from build123d import *

# Parameters (mm, degrees)
SKETCH1_W           = 42
SKETCH1_H           = 42
BOSS_EXTRUDE1_DEPTH = 37.5
SKETCH2_R           = 2.5
BOSS_EXTRUDE2_DEPTH = 23
SKETCH3_R           = 1.5
CUT_EXTRUDE1_DEPTH  = 8
SKETCH4_R           = 11
BOSS_EXTRUDE3_DEPTH = 3
CHAMFER1_SIZE       = 4
SKETCH5_W           = 18
SKETCH5_H           = 10
BOSS_EXTRUDE4_DEPTH = 6
FILLET1_START       = 10
FILLET1_DEPTH       = 19.5
FILLET2_START       = 10
FILLET2_DEPTH       = 19.5
FILLET3_START       = 10
FILLET3_DEPTH       = 19.5


with BuildPart() as part:
    # Sketch1 → Boss-Extrude1 (new body)
    with BuildSketch(Plane(origin=(0, 0, 0), x_dir=(1, 0, 0), z_dir=(0, 1, 0))):
        with Locations((21, 21)):
            Rectangle(SKETCH1_W, SKETCH1_H)
    extrude(amount=BOSS_EXTRUDE1_DEPTH)

    # Sketch2 → Boss-Extrude2 (add)
    with BuildSketch(Plane(origin=(0, 37.5, 0), x_dir=(1, 0, 0), z_dir=(0, 1, 0))):
        with Locations(Location((21, 21, 0), (0, 0, 90))):
            Circle(SKETCH2_R)
    extrude(amount=BOSS_EXTRUDE2_DEPTH)

    # Sketch3 → Cut-Extrude1 (cut)
    with BuildSketch(Plane(origin=(0, 37.5, 0), x_dir=(1, 0, 0), z_dir=(0, 1, 0))):
        with Locations(Location((6, 36, 0), (0, 0, 270))):
            Circle(SKETCH3_R)
        with Locations(Location((36, 36, 0), (0, 0, 270))):
            Circle(SKETCH3_R)
        with Locations(Location((36, 6, 0), (0, 0, 270))):
            Circle(SKETCH3_R)
        with Locations(Location((6, 6, 0), (0, 0, 270))):
            Circle(SKETCH3_R)
    extrude(amount=-CUT_EXTRUDE1_DEPTH, mode=Mode.SUBTRACT)

    # Sketch4 → Boss-Extrude3 (add)
    with BuildSketch(Plane(origin=(0, 37.5, 0), x_dir=(1, 0, 0), z_dir=(0, 1, 0))):
        with Locations(Location((21, 21, 0), (0, 0, 90))):
            Circle(SKETCH4_R)
    extrude(amount=BOSS_EXTRUDE3_DEPTH)

    # Chamfer1
    chamfer1_edges = [part.edges().sort_by_distance(p)[0] for p in [
        (0, 18.75, -42),
        (42, 18.75, -42),
        (42, 18.75, 0),
        (0, 18.75, 0),
    ]]
    chamfer(chamfer1_edges, length=CHAMFER1_SIZE)

    # Sketch5 → Boss-Extrude4 (add)
    with BuildSketch(Plane.ZY):
        with Locations((-21, 5)):
            Rectangle(SKETCH5_W, SKETCH5_H)
    extrude(amount=BOSS_EXTRUDE4_DEPTH)

    # Fillet1: read off the stored shape, not the designer's step
    # Fillet1 outline → Fillet1 (cut)
    with BuildSketch(Plane(origin=(0, 0, 0), x_dir=(1, 0, 0), z_dir=(0, 1, 0)).offset(FILLET1_START)):
        with BuildLine():
            ThreePointArc((42, 6.485281374), (41.543277195, 4.18918078), (40.242640687, 2.242640687))
            Line((40.242640687, 2.242640687), (42, 4))
            Line((42, 4), (42, 6.485281374))
        make_face()
        with BuildLine():
            ThreePointArc((39.757359313, 1.757359313), (37.81081922, 0.456722805), (35.514718626, 0))
            Line((35.514718626, 0), (38, 0))
            Line((38, 0), (39.757359313, 1.757359313))
        make_face()
    extrude(amount=FILLET1_DEPTH, mode=Mode.SUBTRACT)

    # Fillet2: read off the stored shape, not the designer's step
    # Fillet2 outline → Fillet2 (cut)
    with BuildSketch(Plane(origin=(0, 0, 0), x_dir=(1, 0, 0), z_dir=(0, 1, 0)).offset(FILLET2_START)):
        with BuildLine():
            ThreePointArc((35.514718626, 42), (37.81081922, 41.543277195), (39.757359313, 40.242640687))
            Line((39.757359313, 40.242640687), (38, 42))
            Line((38, 42), (35.514718626, 42))
        make_face()
        with BuildLine():
            ThreePointArc((40.242640687, 39.757359313), (41.543277195, 37.81081922), (42, 35.514718626))
            Line((42, 35.514718626), (42, 38))
            Line((42, 38), (40.242640687, 39.757359313))
        make_face()
    extrude(amount=FILLET2_DEPTH, mode=Mode.SUBTRACT)

    # Fillet3: read off the stored shape, not the designer's step
    # Fillet3 outline → Fillet3 (cut)
    with BuildSketch(Plane(origin=(0, 0, 0), x_dir=(1, 0, 0), z_dir=(0, 1, 0)).offset(FILLET3_START)):
        with BuildLine():
            ThreePointArc((6.485281374, 0), (4.18918078, 0.456722805), (2.242640687, 1.757359313))
            Line((2.242640687, 1.757359313), (4, 0))
            Line((4, 0), (6.485281374, 0))
        make_face()
        with BuildLine():
            ThreePointArc((1.757359313, 2.242640687), (0.456722805, 4.18918078), (0, 6.485281374))
            Line((0, 6.485281374), (0, 4))
            Line((0, 4), (1.757359313, 2.242640687))
        make_face()
        with BuildLine():
            ThreePointArc((0, 35.514718626), (0.456722805, 37.81081922), (1.757359313, 39.757359313))
            Line((1.757359313, 39.757359313), (0, 38))
            Line((0, 38), (0, 35.514718626))
        make_face()
        with BuildLine():
            ThreePointArc((2.242640687, 40.242640687), (4.18918078, 41.543277195), (6.485281374, 42))
            Line((6.485281374, 42), (4, 42))
            Line((4, 42), (2.242640687, 40.242640687))
        make_face()
    extrude(amount=FILLET3_DEPTH, mode=Mode.SUBTRACT)


solid = part.part
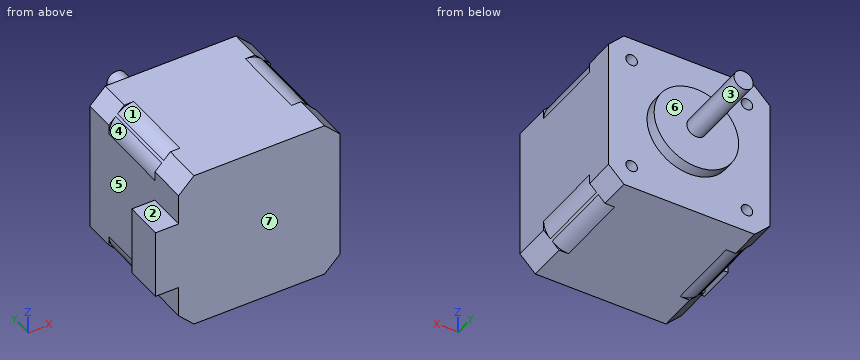
Here's how the part is built. I have some questions about the finished solid (model axes, mm). Face numbers are marked on the shaded views. A direction names the side the tool comes from. Give positions to 0.01 mm unless a question says otherwise; leave off trailing zeros. Loops run counter-clockwise (first coordinate to the right, second up) from the corner with the lowest first, then second, coordinate; pieces in that order, holes last. Notation, with made-up numbers: (-17.5, 79.25) -> (-10.5, 79.25) arc R28 cw to (-10.5, 116.25) -> close; hole circle Ø11 at (70.25, 63). An arc over 180 degrees is marked (long way). Answer as a JSON object with one key per item and string values. Group by question number.
Item 1: Imagine slicing it at A-A on x = 21. Write out the boundary of the cut face in (y, z).
Item 2: Imagine slicing it at B-B on y = 34. Write out the boundary of the cut face in (x, z), then the cut area to 3 significant figures.
Item 3: Imagine slicing it at C-C on z = -21. Write out the boundary of the cut face in (x, y).
Item 4: Thinking about a two-plate mould opening in Y: for the marked faces 4, 5, 6 and 7, which applies, pulls with the +Y half, pulls with the -Y half, needs draft (parallel to the pull), parting line crosses it, or undercut?
Item 5: On a 3-axis mill with a long thin cutter (end or side, diameter ignored), from which of +Z, -Z, +X, -X, +Y, -Y can I reach the whole of each face in a straight line? I mean the marked faces 1, 2 and 3. Say none if no direction works.
Item 6: I need wall thicknesses on L1, parallel to X at y = 32.75, z = -36; L2, parallel to X at y = 24.5, z = -20; L3, parallel to Y at x = 8.5, z = -20. Which ranges of each line are inside material? Lowest first, please.
Item 7: Imagine slicing it at D-D on y = 25. Write out the boundary of the cut face in (x, z), then the cut area to 3 significant figures.
Item 8: Will these pins go through, and if not, where does the flat tip stop? pin 1 (1.9 mm diameter, centred on x = 41.5, z = -38.5, fed in from +Y); pin 2 (21 mm diameter, centred on x = 11.5, z = -10.5, fed in from +Y); pin 3 (1.5 mm diameter, centred on x = 36, z = -36, fed in from +Y); pin 4 (12 mm diameter, centred on x = 12, y = 51, fed in from +Z).
Answer list:
{
 "1": {"outline": "(0, -42) -> (37.5, -42) -> (37.5, -32) -> (40.5, -32) -> (40.5, -23.5) -> (60.5, -23.5) -> (60.5, -18.5) -> (40.5, -18.5) -> (40.5, -10) -> (37.5, -10) -> (37.5, 0) -> (0, 0) -> close"},
 "2": {"outline": "(0, -38) -> (4, -42) -> (38, -42) -> (42, -38) -> (42, -4) -> (38, 0) -> (4, 0) -> (0, -4) -> close; hole circle Ø3 at (6, -36); hole circle Ø3 at (6, -6); hole circle Ø3 at (36, -36); hole circle Ø3 at (36, -6)", "area": "1,700 mm2"},
 "3": {"outline": "(-6, 0) -> (42, 0) -> (42, 37.5) -> (32, 37.5) -> (32, 40.5) -> (23.5, 40.5) -> (23.5, 60.5) -> (18.5, 60.5) -> (18.5, 40.5) -> (10, 40.5) -> (10, 37.5) -> (0, 37.5) -> (0, 10) -> (-6, 10) -> close"},
 "4": {"face 4": "undercut", "face 5": "needs draft", "face 6": "pulls with the +Y half", "face 7": "pulls with the -Y half"},
 "5": {"face 1": "+Z, -X", "face 2": "+Z, -X, +Y, -Y", "face 3": "+Y"},
 "6": {"L1": "x = 0 to 4.5, 7.5 to 34.5, 37.5 to 42", "L2": "x = 0 to 42", "L3": "y = 0 to 37.5"},
 "7": {"outline": "(0, -35.51) arc R6 ccw to (1.76, -39.76) -> (2.24, -40.24) arc R6 ccw to (6.49, -42) -> (35.51, -42) arc R6 ccw to (39.76, -40.24) -> (40.24, -39.76) arc R6 ccw to (42, -35.51) -> (42, -6.49) arc R6 ccw to (40.24, -2.24) -> (39.76, -1.76) arc R6 ccw to (35.51, 0) -> (6.49, 0) arc R6 ccw to (2.24, -1.76) -> (1.76, -2.24) arc R6 ccw to (0, -6.49) -> close", "area": "1,730 mm2"},
 "8": {"pin 1": "stops at y = 37.5", "pin 2": "stops at y = 40.5", "pin 3": "stops at y = 29.5", "pin 4": "passes through"}
}
